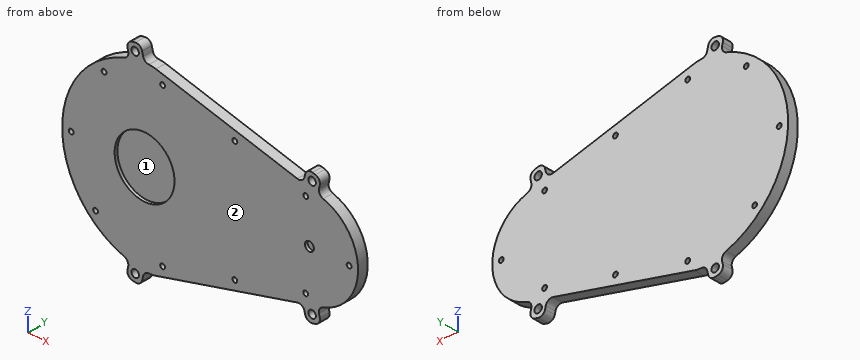
```python
from build123d import *

# Parameters (mm, degrees)
SKETCH1_R           = 1.6
BOSS_EXTRUDE1_DEPTH = 7
BOSS_EXTRUDE2_DEPTH = 7
SKETCH3_R           = 2.5
CUT_EXTRUDE1_DEPTH  = 7
FILLET1_R           = 4
FILLET2_R           = 20
SKETCH5_R           = 20
SKETCH5_R_2         = 3
CUT_EXTRUDE3_DEPTH  = 2


with BuildPart() as part:
    # Sketch1 → Boss-Extrude1 (new body)
    with BuildSketch(Plane(origin=(0, 0, 0), x_dir=(1, 0, 0), z_dir=(0, 1, 0))):
        with BuildLine():
            Line((-40.085587865, -58.991121495), (72.606562154, -30.567708203))
            ThreePointArc((72.606562154, -30.567708203), (97.414412135, 1.008878505), (72.606562154, 32.585465212))
            Line((72.606562154, 32.585465212), (-40.085587865, 61.008878505))
            ThreePointArc((-40.085587865, 61.008878505), (-100.085587865, 1.008878505), (-40.085587865, -58.991121495))
        make_face()
        with Locations(Location((15.176377483, -38.864945804, 0), (0, 0, 270))):
            Circle(SKETCH1_R, mode=Mode.SUBTRACT)
        with Locations(Location((-33.054187001, -51.02974404, 0), (0, 0, 270))):
            Circle(SKETCH1_R, mode=Mode.SUBTRACT)
        with Locations(Location((62.43730848, -26.944710242, 0), (0, 0, 270))):
            Circle(SKETCH1_R, mode=Mode.SUBTRACT)
        with Locations(Location((91.414412135, 1.008878505, 0), (0, 0, 270))):
            Circle(SKETCH1_R, mode=Mode.SUBTRACT)
        with Locations(Location((-33.054187001, 53.047501049, 0), (0, 0, 270))):
            Circle(SKETCH1_R, mode=Mode.SUBTRACT)
        with Locations(Location((15.176377483, 40.882702814, 0), (0, 0, 270))):
            Circle(SKETCH1_R, mode=Mode.SUBTRACT)
        with Locations(Location((62.43730848, 28.962467251, 0), (0, 0, 270))):
            Circle(SKETCH1_R, mode=Mode.SUBTRACT)
        with Locations(Location((-94.085587865, 1.008878505, 0), (0, 0, 270))):
            Circle(SKETCH1_R, mode=Mode.SUBTRACT)
        with Locations(Location((-72.125195915, -42.459081144, 0), (0, 0, 270))):
            Circle(SKETCH1_R, mode=Mode.SUBTRACT)
        with Locations(Location((-77.764180777, 39.691221197, 0), (0, 0, 270))):
            Circle(SKETCH1_R, mode=Mode.SUBTRACT)
    extrude(amount=BOSS_EXTRUDE1_DEPTH)

    # Sketch2 → Boss-Extrude2 (add)
    with BuildSketch(Plane(origin=(0, 7, 0), x_dir=(1, 0, 0), z_dir=(0, 1, 0))):
        Polygon((-55.149276996, 59.087146986), (-45.294016341, 60.782386623), (-47.607258378, 70.511153826), (-57.462519032, 68.815914188), align=None)
        Polygon((60.73773507, 35.579041761), (70.434069941, 33.133415038), (72.769614826, 42.856852192), (63.073279955, 45.302478915), align=None)
        Polygon((63.073279955, -43.284721905), (72.769614826, -40.839095183), (70.434069941, -31.115658029), (60.73773507, -33.561284751), align=None)
        Polygon((-57.462519032, -66.798157179), (-47.607258378, -68.493396816), (-45.294016341, -58.764629614), (-55.149276996, -57.069389977), align=None)
    extrude(amount=-BOSS_EXTRUDE2_DEPTH)

    # Sketch3 → Cut-Extrude1 (cut)
    with BuildSketch(Plane(origin=(0, 7, 0), x_dir=(1, 0, 0), z_dir=(0, 1, 0))):
        with Locations(Location((-51.385785587, 64.787762931, 0), (0, 0, 270))):
            Circle(SKETCH3_R)
        with Locations(Location((66.753288323, 39.217713116, 0), (0, 0, 270))):
            Circle(SKETCH3_R)
        with Locations(Location((66.753288323, -37.199956106, 0), (0, 0, 90))):
            Circle(SKETCH3_R)
        with Locations(Location((-51.385785587, -62.770005922, 0), (0, 0, 90))):
            Circle(SKETCH3_R)
    extrude(amount=-CUT_EXTRUDE1_DEPTH, mode=Mode.SUBTRACT)

    # Fillet1
    fillet1_edges = [part.edges().sort_by_distance(p)[0] for p in [
        (-55.149276996, 3.5, 57.069389977),
        (-57.462519032, 3.5, 66.798157179),
        (-47.607258378, 3.5, 68.493396816),
        (-45.294016341, 3.5, 58.764629614),
        (70.434069941, 3.5, 31.115658029),
        (72.769614826, 3.5, 40.839095183),
        (63.073279955, 3.5, 43.284721905),
        (60.73773507, 3.5, 33.561284751),
        (60.73773507, 3.5, -35.579041761),
        (63.073279955, 3.5, -45.302478915),
        (72.769614826, 3.5, -42.856852192),
        (70.434069941, 3.5, -33.133415038),
        (-45.294016341, 3.5, -60.782386623),
        (-55.149276996, 3.5, -59.087146986),
        (-47.607258378, 3.5, -70.511153826),
        (-57.462519032, 3.5, -68.815914188),
    ]]
    fillet(fillet1_edges, radius=FILLET1_R)

    # Fillet2
    fillet2_edges = [part.edges().sort_by_distance(p)[0] for p in [
        (-40.085587865, 3.5, 58.991121495),
        (-40.085587865, 3.5, -61.008878505),
    ]]
    fillet(fillet2_edges, radius=FILLET2_R)

    # Sketch5 → Cut-Extrude3 (cut)
    with BuildSketch(Plane.XZ):
        with Locations(Location((-45.085587865, -1.008878505, 0), (0, 0, 270))):
            Circle(SKETCH5_R)
        with Locations(Location((64.914412135, -1.008878505, 0), (0, 0, 270))):
            Circle(SKETCH5_R_2)
    extrude(amount=-CUT_EXTRUDE3_DEPTH, mode=Mode.SUBTRACT)


solid = part.part
```
Geometry check sheet. Reference: the model listing, model coordinates, mm. Face numbers are marked on the shaded views. Round coordinates to 2 decimals unless told otherwise and drop trailing zeros. Loops run counter-clockwise (first coordinate to the right, second up) from the corner with the lowest first, then second, coordinate; pieces in that order, holes last. Notation, with made-up numbers: (34, 46) - (87, 46) arc R29 cw to (87, 77) - close; hole circle Ø5 at (70.25, 8.5). An arc over 180 degrees is marked (long way). Write each question's results on one line, items separated by ' | '. Start each with the question number.
Q1. Cross-section at B-B on y = 3.5. State how many separate pieces and enclosed holes the cut face has, and give its area (3 significant figures).
Q2. Thickness scan on line 1 (Y direction, x = -63.5, z = 3); line 2 (Z direction, x = -86.5, y = 0.75); line 3 (Z direction, x = -26, y = 2.25). Record the ranges inside material, lowest first. Write a range as [from, to].
Q3. Cross-section at D-D on z = -6. Enter the section's corners in (x, y), and give its area (3 significant figures).
Q4. Gauge pin test, flat ends, axial feed: P1, Ø4, axis at x = -59.5, y = 2.5, coming from the +Z side (3 decimals); P2, Ø4, axis at y = 1.5, z = 12.5, coming from the +X side; P3, Ø1.5, axis at x = -30.5, y = 4.5, coming from the +Z side. Record the tip position at first contact, or that the pin passes through.
Q5. Release check for a two-part mould opening along Z. For the marked faces 1 and 2 record: +Z half, -Z half, draft (parallel to the pull), parting line (faces both ways), or undercut.
Q6. Cross-section at C-C on x = -20.5. Enter the section's corners in (y, z).
Q7. Cross-section at A-A on z = 11.5. Enter the section's corners in (x, y), and give its area (3 significant figures).
Answers below:
1) separate pieces: 1 | enclosed holes: 14 | area: 17,400 mm²
2) line 1: y = [2, 7] | line 2: z = [-39.03, 37.01] | line 3: z = [-57.46, 55.44]
3) outline: (-99.88, 0) - (-64.45, 0) - (-64.45, 2) - (-25.72, 2) - (-25.72, 0) - (97.03, 0) - (97.03, 7) - (-99.88, 7) - close | area: 1,300 mm²
4) P1: stops at z = 56.655 | P2: stops at x = 95.31 | P3: stops at z = 56.76
5) face 1: undercut | face 2: draft
6) outline: (0, -56.07) - (7, -56.07) - (7, 54.05) - (0, 54.05) - close
7) outline: (-98.77, 0) - (-60.69, 0) - (-60.69, 2) - (-29.48, 2) - (-29.48, 0) - (94.91, 0) - (94.91, 7) - (-98.77, 7) - close | area: 1,290 mm²
